from build123d import *

# Parameters (mm, degrees)
SKETCH1_R                = 47.5
SKETCH1_R_2              = 25
BOSS_EXTRUDE1_DEPTH      = 100
BOSS_EXTRUDE2_REACH      = 797.244
BOSS_EXTRUDE2_END_RADIUS = 47.5
SKETCH2_R                = 25
SKETCH3_R                = 40
BOSS_EXTRUDE3_DEPTH      = 50


with BuildPart() as part:
    # Sketch1 → Boss-Extrude1 (new body)
    with BuildSketch(Plane.XY):
        Circle(SKETCH1_R)
        Circle(SKETCH1_R_2, mode=Mode.SUBTRACT)
    extrude(amount=BOSS_EXTRUDE1_DEPTH)

    # Boss-Extrude2: up to this cylinder (the profile starts outside it)
    boss_extrude2_end = Plane(origin=(0, 0, 50), z_dir=(0, 0, -1)) * Cylinder(BOSS_EXTRUDE2_END_RADIUS, 1690.488, mode=Mode.PRIVATE)
    # Sketch2 → Boss-Extrude2 (add, up to the surface)
    with BuildSketch(Plane(origin=(740, 0, 0), x_dir=(0, 0, -1), z_dir=(1, 0, 0)), mode=Mode.PRIVATE) as boss_extrude2_sk1:
        with Locations((-50, 0)):
            Circle(SKETCH2_R)
    boss_extrude2_tool1 = extrude(boss_extrude2_sk1.sketch, amount=-BOSS_EXTRUDE2_REACH, mode=Mode.PRIVATE) - boss_extrude2_end
    add(boss_extrude2_tool1.solids().sort_by_distance((740, 0, 50))[0])

    # Sketch3 → Boss-Extrude3 (add)
    with BuildSketch(Plane(origin=(740, 0, 0), x_dir=(0, 0, -1), z_dir=(1, 0, 0))):
        with Locations((-50, 0)):
            Circle(SKETCH3_R)
    extrude(amount=-BOSS_EXTRUDE3_DEPTH)


solid = part.part
The model under review builds one solid part; all positions refer to its coordinate system, in mm. A direction names the side the tool comes from. Give positions to 0.01 mm unless a question says otherwise; leave off trailing zeros. Order: outer loops, then holes, each group sorted by start corner. A loop starts at its lowest first (then second) coordinate and runs counter-clockwise, first axis right, second up. Notation, with made-up numbers: (48, 16) -> (80, 16) arc R26 cw to (80, 33) -> close; hole circle Ø10 at (89.25, 87). An arc over 180 degrees is marked (long way). Write item = value, one per line. Start each with the question number.
(1) Take a section at C-C (z = 50). Write out the cut boundary in (x, y).
(2) Take a section at A-A (x = 0). Write out the cut boundary in (y, z), plus the area to 3 significant figures.
(3) For L1, parallel to Y at x = 0, z = 69.5; L2, parallel to X at y = 8, z = 23; L3, parallel to Z at x = 321.5, y = 2, list the stretches that pass through material, from the lowest coordinate up. Write a range as from..to.
(4) Tool access review of faces 4 (the flat face through (20, -20, 100)), 5 (the cylindrical face through (370, -15, 70)), 6 (the cylindrical face through (715.35, 12.015, 11.847)): name each direction out of +Z, -Z, +X, -X, +Y, -Y from which nothing blocks a thin tool from reaching the whole face with its end or side.
(5) Take a section at D-D (x = 254). Write out the cut boundary in (y, z), plus the area to 3 significant figures.
(6) For pin 1 Ø3 at (x, z) = (632, 23) entering from +Y; pin 2 Ø2 at (x, z) = (436, 55.5) entering from +Y; pin 3 Ø5 at (x, z) = (421, 34.5) entering from +Y; pin 4 Ø1 at (x, z) = (535.5, 62.5) entering from +Y, all flat-tipped, find the tip position at first contact; note any pin that passes through.
(7) Draft analysis for pull direction X (two halves, no side actions). For faces 1 (the flat face through (690, 18.34, 32.78)), 2 (the flat face through (20, -20, 0)), 3 (the flat face through (740, 1, 51)), state which applies: +X half, -X half, draft (parallel to the pull), parting line (faces both ways), or undercut.
(8) Take a section at B-B (y = 0). Write out the cut boundary in (x, z).
Returned:
q1.outline = (40.39, -25) -> (690, -25) -> (690, -40) -> (740, -40) -> (740, 40) -> (690, 40) -> (690, 25) -> (40.39, 25) arc R47.5 ccw (long way) to start; hole circle Ø50 at (0, 0)
q2.outline = (-47.5, 0) -> (-25, 0) -> (-25, 100) -> (-47.5, 100) -> close; (25, 0) -> (47.5, 0) -> (47.5, 100) -> (25, 100) -> close
q2.area = 4,500 mm²
q3.L1 = -47.5..-25, 25..47.5
q3.L2 = -46.82..-23.69, 23.69..46.82, 690..740
q3.L3 = 25.08..74.92
q4.face_4 = +Z, +X, -X, +Y, -Y
q4.face_5 = none
q4.face_6 = +X
q5.outline = circle Ø50 at (0, 50)
q5.area = 1,960 mm²
q6.pin_1 = through
q6.pin_2 = 24.59
q6.pin_3 = 21.35
q6.pin_4 = 21.93
q7.face_1 = undercut
q7.face_2 = draft
q7.face_3 = +X half
q8.outline = (-47.5, 0) -> (-25, 0) -> (-25, 100) -> (-47.5, 100) -> close; (25, 0) -> (47.5, 0) -> (47.5, 25) -> (690, 25) -> (690, 10) -> (740, 10) -> (740, 90) -> (690, 90) -> (690, 75) -> (47.5, 75) -> (47.5, 100) -> (25, 100) -> close
